```python
from build123d import *

# Parameters (mm, degrees)
BOSS_EXTRUDE1_DEPTH = 2.25
FILLET1_R           = 5
SKETCH2_R           = 1.75
CUT_EXTRUDE1_DEPTH  = 45.881363874
BOSS_EXTRUDE2_REACH = 39.627
SKETCH4_W           = 6
SKETCH4_H           = 2.1
SKETCH4_2_W         = 6
SKETCH4_2_H         = 2.1
BOSS_EXTRUDE3_DEPTH = 2.150401339
FILLET2_R           = 3
FILLET3_R           = 1.2
FILLET4_R           = 0.5


with BuildPart() as part:
    # Sketch1 → Boss-Extrude1 (new body)
    with BuildSketch(Plane(origin=(0, 0, 0), x_dir=(1, 0, 0), z_dir=(0, 1, 0))):
        Polygon((0, 0), (9.481214188, 15.300541739), (16.403607864, 39.323040897), (21.51680222, 39.323040897), (17.140904697, 12.99204844), (7.659690509, -2.308493299), align=None)
    extrude(amount=BOSS_EXTRUDE1_DEPTH)

    # Fillet1
    # the kernel refuses this fillet: 5 mm, written as the material it takes off along each edge
    with BuildSketch(Plane(origin=(7.659690509, -9.589301146, 2.308493299), x_dir=(0.5267341215597666, 0, -0.8500300966346198), z_dir=(0, 1, 0))) as fillet1_piece_1:
        with BuildLine():
            CenterArc((FILLET1_R * 0.767144091705, FILLET1_R), FILLET1_R, 195.013192562, 74.986807438)
            Line((-FILLET1_R * 0.19872211495, FILLET1_R * 0.740958553812), (0, 0))
            Line((0, 0), (FILLET1_R * 0.767144091705, 0))
        make_face()
    extrude(amount=21.428602293, mode=Mode.SUBTRACT)
    with BuildSketch(Plane(origin=(0, -16.294200966, 0), x_dir=(0.5267341215597675, 0, -0.8500300966346193), z_dir=(0, 1, 0))) as fillet1_piece_2:
        with BuildLine():
            CenterArc((FILLET1_R * 1.30353607727, -FILLET1_R), FILLET1_R, 90, 105.013192562)
            Line((FILLET1_R * 0.337669870614, -FILLET1_R * 1.25904144619), (0, 0))
            Line((0, 0), (FILLET1_R * 1.30353607727, 0))
        make_face()
    extrude(amount=34.838401932, mode=Mode.SUBTRACT)

    # Sketch2 → Cut-Extrude1 (cut, through all)
    with BuildSketch(Plane(origin=(0, 2.25, 0), x_dir=(1, 0, 0), z_dir=(0, 1, 0))):
        with Locations(Location((8.167211871, 5.629873064, 0), (0, 0, 270))):
            Circle(SKETCH2_R)
        with Locations(Location((13.979207558, 18.366462331, 0), (0, 0, 270))):
            Circle(SKETCH2_R)
    extrude(amount=-CUT_EXTRUDE1_DEPTH, mode=Mode.SUBTRACT)

    # Boss-Extrude2: up to this plane
    boss_extrude2_end = Plane(origin=(17.140904697, 2.25, -12.99204844), z_dir=(-0.9864703728289792, 0, -0.16393963380053925))
    # Sketch4 → Boss-Extrude2 (add, up to the surface)
    with BuildSketch(Plane(origin=(23.5, -1.484709168, -8.201879583), x_dir=(0, 0, -1), z_dir=(1, 0, 0)), mode=Mode.PRIVATE) as boss_extrude2_sk1:
        with Locations((27.115050996, 2.541926215)):
            Rectangle(SKETCH4_W, SKETCH4_H)
    boss_extrude2_tool1 = split(extrude(boss_extrude2_sk1.sketch, amount=-BOSS_EXTRUDE2_REACH, mode=Mode.PRIVATE), bisect_by=boss_extrude2_end, keep=Keep.BOTH, mode=Mode.PRIVATE)
    add(boss_extrude2_tool1.solids().sort_by_distance((23.5, 1.057217, -35.316931))[0])

    # Sketch4<2> → Boss-Extrude3 (add)
    with BuildSketch(Plane(origin=(23.5, -1.484709168, -8.201879583), x_dir=(0, 0, -1), z_dir=(1, 0, 0))):
        with Locations((27.115050996, 2.541926215)):
            Rectangle(SKETCH4_2_W, SKETCH4_2_H)
    extrude(amount=-BOSS_EXTRUDE3_DEPTH)

    # Fillet2
    fillet2_edges = [part.edges().sort_by_distance(p)[0] for p in [
        (16.403607864, 1.125, -39.323040897),
    ]]
    fillet(fillet2_edges, radius=FILLET2_R)

    # Fillet3
    # the kernel refuses this fillet: 1.2 mm, written as the material it takes off along each edge
    with BuildSketch(Plane(origin=(21.51680222, -3.539709856, -39.323040897), x_dir=(-1, 0, 0), z_dir=(0, 1, 0))) as fillet3_piece_1_section:
        with BuildLine():
            CenterArc((FILLET3_R * 1.17990328535, FILLET3_R), FILLET3_R, 170.564358813, 99.435641187)
            Line((FILLET3_R * 0.19343291252, FILLET3_R * 1.1639396338), (0, 0))
            Line((0, 0), (FILLET3_R * 1.17990328535, 0))
        make_face()
    fillet3_piece_1 = extrude(amount=9.329419712, mode=Mode.PRIVATE)
    fillet3_piece_1 = split(fillet3_piece_1, bisect_by=Plane(origin=(21.129198659, 0.007217047, -39.030141568), z_dir=(0, -1, 0)), keep=Keep.TOP, mode=Mode.PRIVATE)
    fillet3_piece_1 = split(fillet3_piece_1, bisect_by=Plane(origin=(21.129198659, -1.766246404, -38.316930579), z_dir=(0, 0, -1)), keep=Keep.TOP, mode=Mode.PRIVATE)
    add(fillet3_piece_1, mode=Mode.SUBTRACT)
    with BuildSketch(Plane(origin=(21.51680222, -3.539709856, -39.323040897), x_dir=(-1, 0, 0), z_dir=(0, 1, 0))) as fillet3_piece_2_section:
        with BuildLine():
            CenterArc((FILLET3_R * 1.17990328535, FILLET3_R), FILLET3_R, 170.564358813, 99.435641187)
            Line((FILLET3_R * 0.19343291252, FILLET3_R * 1.1639396338), (0, 0))
            Line((0, 0), (FILLET3_R * 1.17990328535, 0))
        make_face()
    fillet3_piece_2 = extrude(amount=9.329419712, mode=Mode.PRIVATE)
    fillet3_piece_2 = split(fillet3_piece_2, bisect_by=Plane(origin=(21.322056941, 0.007217047, -38.16671154), z_dir=(0, -1, 0)), keep=Keep.TOP, mode=Mode.PRIVATE)
    fillet3_piece_2 = split(fillet3_piece_2, bisect_by=Plane(origin=(21.322056941, -1.766246404, -38.316930579), z_dir=(0, 0, 1)), keep=Keep.TOP, mode=Mode.PRIVATE)
    add(fillet3_piece_2, mode=Mode.SUBTRACT)
    with BuildSketch(Plane(origin=(21.51680222, -3.539709856, -39.323040897), x_dir=(-1, 0, 0), z_dir=(0, 1, 0))) as fillet3_piece_3_section:
        with BuildLine():
            CenterArc((FILLET3_R * 1.17990328535, FILLET3_R), FILLET3_R, 170.564358813, 99.435641187)
            Line((FILLET3_R * 0.19343291252, FILLET3_R * 1.1639396338), (0, 0))
            Line((0, 0), (FILLET3_R * 1.17990328535, 0))
        make_face()
    fillet3_piece_3 = extrude(amount=9.329419712, mode=Mode.PRIVATE)
    fillet3_piece_3 = split(fillet3_piece_3, bisect_by=Plane(origin=(21.129198659, 2.107217047, -39.030141568), z_dir=(0, -1, 0)), keep=Keep.TOP, mode=Mode.PRIVATE)
    fillet3_piece_3 = split(fillet3_piece_3, bisect_by=Plane(origin=(21.129198659, 0.007217047, -39.030141568), z_dir=(0, 1, 0)), keep=Keep.TOP, mode=Mode.PRIVATE)
    fillet3_piece_3 = split(fillet3_piece_3, bisect_by=Plane(origin=(21.129198659, 1.057217047, -38.316930579), z_dir=(0, 0, -1)), keep=Keep.TOP, mode=Mode.PRIVATE)
    add(fillet3_piece_3, mode=Mode.SUBTRACT)
    with BuildSketch(Plane(origin=(21.51680222, -3.539709856, -39.323040897), x_dir=(-1, 0, 0), z_dir=(0, 1, 0))) as fillet3_piece_4_section:
        with BuildLine():
            CenterArc((FILLET3_R * 1.17990328535, FILLET3_R), FILLET3_R, 170.564358813, 99.435641187)
            Line((FILLET3_R * 0.19343291252, FILLET3_R * 1.1639396338), (0, 0))
            Line((0, 0), (FILLET3_R * 1.17990328535, 0))
        make_face()
    fillet3_piece_4 = extrude(amount=9.329419712, mode=Mode.PRIVATE)
    fillet3_piece_4 = split(fillet3_piece_4, bisect_by=Plane(origin=(21.129198659, 2.107217047, -39.030141568), z_dir=(0, 1, 0)), keep=Keep.TOP, mode=Mode.PRIVATE)
    fillet3_piece_4 = split(fillet3_piece_4, bisect_by=Plane(origin=(21.129198659, 3.948463452, -38.316930579), z_dir=(0, 0, -1)), keep=Keep.TOP, mode=Mode.PRIVATE)
    add(fillet3_piece_4, mode=Mode.SUBTRACT)
    with BuildSketch(Plane(origin=(21.51680222, -3.539709856, -39.323040897), x_dir=(-1, 0, 0), z_dir=(0, 1, 0))) as fillet3_piece_5_section:
        with BuildLine():
            CenterArc((FILLET3_R * 1.17990328535, FILLET3_R), FILLET3_R, 170.564358813, 99.435641187)
            Line((FILLET3_R * 0.19343291252, FILLET3_R * 1.1639396338), (0, 0))
            Line((0, 0), (FILLET3_R * 1.17990328535, 0))
        make_face()
    fillet3_piece_5 = extrude(amount=9.329419712, mode=Mode.PRIVATE)
    fillet3_piece_5 = split(fillet3_piece_5, bisect_by=Plane(origin=(21.322056941, 2.107217047, -38.16671154), z_dir=(0, 1, 0)), keep=Keep.TOP, mode=Mode.PRIVATE)
    fillet3_piece_5 = split(fillet3_piece_5, bisect_by=Plane(origin=(21.322056941, 3.948463452, -38.316930579), z_dir=(0, 0, 1)), keep=Keep.TOP, mode=Mode.PRIVATE)
    add(fillet3_piece_5, mode=Mode.SUBTRACT)

    # Fillet4
    fillet4_edges = [part.edges().sort_by_distance(p)[0] for p in [
        (23.5, 1.057217047, -38.316930579),
        (23.5, 1.057217047, -32.316930579),
    ]]
    fillet(fillet4_edges, radius=FILLET4_R)


solid = part.part
```
Model file for the job. Use its own axes, mm. A direction names the side the tool comes from. Give positions to 0.01 mm unless a question says otherwise; leave off trailing zeros. Order: outer loops, then holes, each group sorted by start corner. A loop starts at its lowest first (then second) coordinate and runs counter-clockwise, first axis right, second up.
1) Saw through at C-C, the plane y = 0.8. Write the cut outline in (x, z).
2) Wall check: probe 1 along Z at (x, y) = (22.25, 1.1); probe 2 along Z at (x, y) = (7, 1.1); probe 3 along Z at (x, y) = (8.25, 1.05). Give the ranges that are in metal, low to high.
3) Saw through at A-A, the plane x = 15. Write the cut outline in (y, z), then the cut area to 3 significant figures.
4) Pin check, flat tips, straight feed: pin 1 (0.6 mm diameter, centred on x = 21, y = 1, fed in from +Z); pin 2 (1 mm diameter, centred on y = 0.5, z = -20, fed in from +X); pin 3 (10 mm diameter, centred on x = 5.5, z = -31, fed in from +Y); pin 4 (0.5 mm diameter, centred on x = 22, y = 1.5, fed in from -Z). Stop position of each tip, or through.
5) Mould opens along X. For faces 1 (the flat face through (22, 2.107, -35)), 2 (the flat face through (12.586, 1.109, -26.074)), 3 (the cylindrical face through (9.9, 1.14, -5.86)) say: +X half, -X half, draft (parallel to the pull), parting line (faces both ways), or undercut.
6) Saw through at B-B, the plane z = -18. Write the cut outline in (x, y), then the cut area to 3 significant figures.
7) 3-axis set-ups, long thin cutter, end or side, ignore diameter. For faces 4 (the flat face through (12, 0, -19)), 5 (the flat face through (22, 1, -32.317)), 6 (the flat face through (22, 1, -38.317)): which of +Z, -Z, +X, -X, +Y, -Y reach the whole face in a straight line?
8) Saw through at D-D, the plane z = -8. Write the cut outline in (x, y).
Computed:
1. outline: (3.43, -5.54) - (9.48, -15.3) - (15.78, -37.15) arc R3 ccw to (18.66, -39.32) - (20.1, -39.32) arc R1.2 ccw to (21.29, -38.32) - (23, -38.32) arc R0.5 ccw to (23.5, -37.82) - (23.5, -32.82) arc R0.5 ccw to (23, -32.32) - (20.35, -32.32) - (17.14, -12.99) - (9.68, -0.95) arc R5 ccw to (5.15, 1.41) arc R5 ccw to start; hole circle Ø3.5 at (8.17, -5.63); hole circle Ø3.5 at (13.98, -18.37)
2. probe 1: z = -38.32 to -32.32
2. probe 2: z = -11.3 to -6.93, -4.33 to 1.16
2. probe 3: z = -13.31 to -7.38, -3.88 to 0.54
3. outline: (0, -34.45) - (2.25, -34.45) - (2.25, -19.79) - (0, -19.79) - close; (0, -16.95) - (2.25, -16.95) - (2.25, -9.54) - (0, -9.54) - close
3. area: 49.7 mm2
4. pin 1: stops at z = -32.32
4. pin 2: stops at x = 18.39
4. pin 3: passes through
4. pin 4: stops at z = -38.32
5. face 1: draft
5. face 2: -X half
5. face 3: undercut
6. outline: (10.26, 0) - (12.27, 0) - (12.27, 2.25) - (10.26, 2.25) - close; (15.69, 0) - (17.97, 0) - (17.97, 2.25) - (15.69, 2.25) - close
6. area: 9.66 mm2
7. face 4: +Z, -Z, +X, -X, -Y
7. face 5: +Z, +X, +Y, -Y
7. face 6: -Z, +X, +Y, -Y
8. outline: (4.96, 0) - (14.05, 0) - (14.05, 2.25) - (4.96, 2.25) - close
